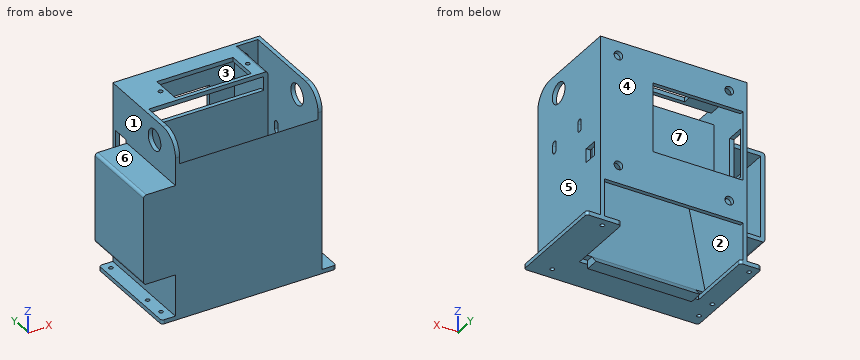
from build123d import *

# Parameters (mm, degrees)
SKETCH_1_W                      = 126
SKETCH_1_H                      = 75
EXTRUDE_1_DEPTH                 = 3
CUT_EXTRUDE_2_REACH             = 148.663
SKETCH_3_W                      = 86
SKETCH_3_H                      = 50
SKETCH_2_R                      = 1.5
CUT_EXTRUDE_1_DEPTH             = 147.662878739
SKETCH_4_W                      = 3
SKETCH_4_H                      = 75
EXTRUDE_2_DEPTH                 = 130
SKETCH_10_W                     = 100
SKETCH_10_H                     = 3
EXTRUDE_5_DEPTH                 = 100
CUT_EXTRUDE_5_REACH             = 199.965
SKETCH_9_R                      = 3.1
CUT_EXTRUDE_5_DIRECTION_2_DEPTH = 198.964643308
EXTRUDE_7_REACH                 = 191.955
CUT_EXTRUDE_9_DEPTH             = 190.95525789
CUT_EXTRUDE_9_DEPTH_BACK        = 190.95525789
SKETCH_18_R                     = 7.55
SKETCH_33_W                     = 65
SKETCH_33_H                     = 50
CUT_EXTRUDE_14_DEPTH            = 5
FILLET_1_R                      = 2
FILLET_2_R                      = 15
CUT_EXTRUDE_11_DEPTH            = 10
SKETCH_37_W                     = 89
SKETCH_37_H                     = 75
SKETCH_37_W_2                   = 83
SKETCH_37_H_2                   = 69
EXTRUDE_21_DEPTH                = 35
EXTRUDE_22_REACH                = 191.955
SKETCH_38_W                     = 59
SKETCH_38_H                     = 3
EXTRUDE_START                   = 5
EXTRUDE_23_DEPTH                = 75
SKETCH_43_W                     = 65
SKETCH_43_H                     = 58
EXTRUDE_24_DEPTH                = 23
SKETCH_44_W                     = 20
SKETCH_44_H                     = 59
CUT_EXTRUDE_15_DEPTH            = 55
SKETCH_48_W                     = 35
SKETCH_48_H                     = 13
CUT_EXTRUDE_16_DEPTH            = 12
SKETCH_49_W                     = 55
SKETCH_49_H                     = 22
CUT_EXTRUDE_18_DEPTH            = 12
SKETCH_50_R                     = 1.6
SKETCH_50_R_2                   = 1.5
CUT_EXTRUDE_19_DEPTH            = 12
CUT_EXTRUDE_21_REACH            = 201.887
SKETCH_52_W                     = 10
SKETCH_52_H                     = 10
FILLET_3_R                      = 2
SKETCH_53_W                     = 100
SKETCH_53_H                     = 3
EXTRUDE_25_DEPTH                = 3


with BuildPart() as part:
    # 草图1 → 凸台-拉伸1 (new body)
    with BuildSketch(Plane.XY):
        with Locations((63, 37.5)):
            Rectangle(SKETCH_1_W, SKETCH_1_H)
    extrude(amount=EXTRUDE_1_DEPTH)

    # 草图3 → 切除-拉伸2 (cut, up to next)
    with BuildSketch(Plane(origin=(0, 0, 0), x_dir=(-1, 0, 0), z_dir=(0, 0, -1)), mode=Mode.PRIVATE) as cut_extrude_2_sk1:
        with Locations((-58, 50)):
            Rectangle(SKETCH_3_W, SKETCH_3_H)
    cut_extrude_2_tool1 = extrude(cut_extrude_2_sk1.sketch, amount=-CUT_EXTRUDE_2_REACH, mode=Mode.PRIVATE) & part.part
    add(cut_extrude_2_tool1.solids().sort_by_distance((58, 50, 0))[0], mode=Mode.SUBTRACT)

    # 草图2 → 切除-拉伸1 (cut, through all)
    with BuildSketch(Plane.XY.offset(3)):
        with Locations((5, 69)):
            Circle(SKETCH_2_R)
        with Locations((5, 25)):
            Circle(SKETCH_2_R)
        with Locations((5, 9)):
            Circle(SKETCH_2_R)
        with Locations((111, 69)):
            Circle(SKETCH_2_R)
        with Locations((111, 9)):
            Circle(SKETCH_2_R)
    extrude(amount=-CUT_EXTRUDE_1_DEPTH, mode=Mode.SUBTRACT)

    # 草图4 → 凸台-拉伸2 (add)
    with BuildSketch(Plane.XY.offset(3)):
        with Locations((11.5, 37.5)):
            Rectangle(SKETCH_4_W, SKETCH_4_H)
    extrude_2 = extrude(amount=EXTRUDE_2_DEPTH)

    # 镜向1: 凸台-拉伸2 across plane
    add(extrude_2.mirror(Plane.ZY.offset(-63)))

    # 草图10 → 凸台-拉伸5 (add)
    with BuildSketch(Plane(origin=(13, 0, 0), x_dir=(0, 0, -1), z_dir=(1, 0, 0))):
        with Locations((-83, 73.5)):
            Rectangle(SKETCH_10_W, SKETCH_10_H)
    extrude(amount=EXTRUDE_5_DEPTH)

    # 草图9 → 切除-拉伸5 (cut, up to next)
    with BuildSketch(Plane(origin=(0, 75, 0), x_dir=(1, 0, 0), z_dir=(0, 1, 0)), mode=Mode.PRIVATE) as cut_extrude_5_sk1:
        with Locations(Location((23, -123, 0), (0, 0, 180))):
            Circle(SKETCH_9_R)
    cut_extrude_5_tool1 = extrude(cut_extrude_5_sk1.sketch, amount=-CUT_EXTRUDE_5_REACH, mode=Mode.PRIVATE) & part.part
    # 草图9 → 切除-拉伸5 (cut, up to next)
    with BuildSketch(Plane(origin=(0, 75, 0), x_dir=(1, 0, 0), z_dir=(0, 1, 0)), mode=Mode.PRIVATE) as cut_extrude_5_sk2:
        with Locations(Location((23, -43, 0), (0, 0, 180))):
            Circle(SKETCH_9_R)
    cut_extrude_5_tool2 = extrude(cut_extrude_5_sk2.sketch, amount=-CUT_EXTRUDE_5_REACH, mode=Mode.PRIVATE) & part.part
    # 草图9 → 切除-拉伸5 (cut, up to next)
    with BuildSketch(Plane(origin=(0, 75, 0), x_dir=(1, 0, 0), z_dir=(0, 1, 0)), mode=Mode.PRIVATE) as cut_extrude_5_sk3:
        with Locations(Location((103, -123, 0), (0, 0, 180))):
            Circle(SKETCH_9_R)
    cut_extrude_5_tool3 = extrude(cut_extrude_5_sk3.sketch, amount=-CUT_EXTRUDE_5_REACH, mode=Mode.PRIVATE) & part.part
    # 草图9 → 切除-拉伸5 (cut, up to next)
    with BuildSketch(Plane(origin=(0, 75, 0), x_dir=(1, 0, 0), z_dir=(0, 1, 0)), mode=Mode.PRIVATE) as cut_extrude_5_sk4:
        with Locations(Location((103, -43, 0), (0, 0, 180))):
            Circle(SKETCH_9_R)
    cut_extrude_5_tool4 = extrude(cut_extrude_5_sk4.sketch, amount=-CUT_EXTRUDE_5_REACH, mode=Mode.PRIVATE) & part.part
    add(cut_extrude_5_tool1.solids().sort_by_distance((23, 75, 123))[0], mode=Mode.SUBTRACT)
    add(cut_extrude_5_tool2.solids().sort_by_distance((23, 75, 43))[0], mode=Mode.SUBTRACT)
    add(cut_extrude_5_tool3.solids().sort_by_distance((103, 75, 123))[0], mode=Mode.SUBTRACT)
    add(cut_extrude_5_tool4.solids().sort_by_distance((103, 75, 43))[0], mode=Mode.SUBTRACT)

    # 草图9 → 切除-拉伸5 direction 2 (cut)
    with BuildSketch(Plane(origin=(0, 75, 0), x_dir=(1, 0, 0), z_dir=(0, 1, 0))):
        with Locations(Location((23, -123, 0), (0, 0, 180))):
            Circle(SKETCH_9_R)
        with Locations(Location((23, -43, 0), (0, 0, 180))):
            Circle(SKETCH_9_R)
        with Locations(Location((103, -123, 0), (0, 0, 180))):
            Circle(SKETCH_9_R)
        with Locations(Location((103, -43, 0), (0, 0, 180))):
            Circle(SKETCH_9_R)
    extrude(amount=CUT_EXTRUDE_5_DIRECTION_2_DEPTH, mode=Mode.SUBTRACT)

    # 凸台-拉伸7: up to this face of the body (flat: up to its plane)
    extrude_7_end = Plane(part.part.faces().sort_by_distance((113, 36.357142857, 67.523809524))[0])
    # 草图17 → 凸台-拉伸7 (add, up to the picked face)
    with BuildSketch(Plane(origin=(13, 0, 0), x_dir=(0, 0, -1), z_dir=(1, 0, 0)), mode=Mode.PRIVATE) as extrude_7_sk1:
        Polygon((-3, 0), (-113, 0), (-3, 30), align=None)
    extrude_7_tool1 = split(extrude(extrude_7_sk1.sketch, amount=EXTRUDE_7_REACH, mode=Mode.PRIVATE), bisect_by=extrude_7_end, keep=Keep.BOTH, mode=Mode.PRIVATE)
    add(extrude_7_tool1.solids().sort_by(Axis((13, 10, 39.666667), (1, 0, 0)))[0])

    # 草图18 → 切除-拉伸9 (cut, two sides: drawn at the far end of the back side and taken through both)
    with BuildSketch(Plane(origin=(13, 0, 0), x_dir=(0, 0, -1), z_dir=(1, 0, 0)).offset(-CUT_EXTRUDE_9_DEPTH_BACK)):
        with Locations(Location((-118, 25, 0), (0, 0, 90))):
            Circle(SKETCH_18_R)
    extrude(amount=CUT_EXTRUDE_9_DEPTH + CUT_EXTRUDE_9_DEPTH_BACK, mode=Mode.SUBTRACT)

    # 草图33 → 切除-拉伸14 (cut)
    with BuildSketch(Plane(origin=(0, 75, 0), x_dir=(1, 0, 0), z_dir=(0, 1, 0))):
        with Locations((45.5, -86)):
            Rectangle(SKETCH_33_W, SKETCH_33_H)
    extrude(amount=-CUT_EXTRUDE_14_DEPTH, mode=Mode.SUBTRACT)

    # 圆角1
    fillet_1_edges = [part.edges().sort_by_distance(p)[0] for p in [
        (101, 75, 1.5),
        (15, 75, 1.5),
        (0, 0, 1.5),
        (0, 75, 1.5),
        (126, 75, 1.5),
        (126, 0, 1.5),
    ]]
    fillet(fillet_1_edges, radius=FILLET_1_R)

    # 圆角2
    fillet_2_edges = [part.edges().sort_by_distance(p)[0] for p in [
        (11.5, 0, 133),
        (114.5, 0, 133),
    ]]
    fillet(fillet_2_edges, radius=FILLET_2_R)

    # 草图20 → 切除-拉伸11 (cut)
    with BuildSketch(Plane(origin=(116, 0, 0), x_dir=(0, 0, -1), z_dir=(1, 0, 0))):
        with BuildLine():
            Line((-83.606081957, 51.95), (-78.606081957, 51.95))
            ThreePointArc((-78.606081957, 51.95), (-76.556081957, 49.9), (-78.606081957, 47.85))
            Line((-78.606081957, 47.85), (-83.606081957, 47.85))
            ThreePointArc((-83.606081957, 47.85), (-85.656081957, 49.9), (-83.606081957, 51.95))
        make_face()
        with BuildLine():
            Line((-83.606081957, 21.95), (-78.606081957, 21.95))
            ThreePointArc((-78.606081957, 21.95), (-76.556081957, 19.9), (-78.606081957, 17.85))
            Line((-78.606081957, 17.85), (-83.606081957, 17.85))
            ThreePointArc((-83.606081957, 17.85), (-85.656081957, 19.9), (-83.606081957, 21.95))
        make_face()
    extrude(amount=-CUT_EXTRUDE_11_DEPTH, mode=Mode.SUBTRACT)

    # 草图37 → 凸台-拉伸21 (add)
    with BuildSketch(Plane.XZ.offset(-72)):
        with Locations((54.5, 95.5)):
            Rectangle(SKETCH_37_W, SKETCH_37_H)
        with Locations((54.5, 95.5)):
            Rectangle(SKETCH_37_W_2, SKETCH_37_H_2, mode=Mode.SUBTRACT)
    extrude(amount=EXTRUDE_21_DEPTH)

    # 草图38 → 凸台-拉伸22 (add, up to next)
    with BuildSketch(Plane(origin=(13, 0, 0), x_dir=(0, 0, -1), z_dir=(1, 0, 0)), mode=Mode.PRIVATE) as extrude_22_sk1:
        with Locations((-90.5, 38.5)):
            Rectangle(SKETCH_38_W, SKETCH_38_H)
    extrude_22_tool1 = extrude(extrude_22_sk1.sketch, amount=EXTRUDE_22_REACH, mode=Mode.PRIVATE) - part.part
    add(extrude_22_tool1.solids().sort_by_distance((13, 38.5, 90.5))[0])

    # 草图41 → 凸台-拉伸23 (add)
    with BuildSketch(Plane(origin=(15, 0, 0), x_dir=(0, 0, -1), z_dir=(1, 0, 0)).offset(EXTRUDE_START)):
        Polygon((-3, 25), (-3, 30), (3, 35), (3, 25), align=None)
    extrude(amount=EXTRUDE_23_DEPTH)

    # 草图43 → 凸台-拉伸24 (add)
    with BuildSketch(Plane.ZY.offset(-10)):
        with Locations((65.5, 29)):
            Rectangle(SKETCH_43_W, SKETCH_43_H)
    extrude(amount=EXTRUDE_24_DEPTH)

    # 草图44 → 切除-拉伸15 (cut)
    with BuildSketch(Plane(origin=(0, 58, 0), x_dir=(1, 0, 0), z_dir=(0, 1, 0))):
        with Locations((0, -65.5)):
            Rectangle(SKETCH_44_W, SKETCH_44_H)
    extrude(amount=-CUT_EXTRUDE_15_DEPTH, mode=Mode.SUBTRACT)

    # 草图48 → 切除-拉伸16 (cut)
    with BuildSketch(Plane.ZY.offset(-10)):
        with Locations((82.5, 65.5)):
            Rectangle(SKETCH_48_W, SKETCH_48_H)
    extrude(amount=-CUT_EXTRUDE_16_DEPTH, mode=Mode.SUBTRACT)

    # 草图49 → 切除-拉伸18 (cut)
    with BuildSketch(Plane.XY.offset(133)):
        with Locations((61.5, 51)):
            Rectangle(SKETCH_49_W, SKETCH_49_H)
    extrude(amount=-CUT_EXTRUDE_18_DEPTH, mode=Mode.SUBTRACT)

    # 草图50 → 切除-拉伸19 (cut)
    with BuildSketch(Plane.XY.offset(133)):
        with Locations((30, 51)):
            Circle(SKETCH_50_R)
        with Locations((93, 51)):
            Circle(SKETCH_50_R_2)
    extrude(amount=-CUT_EXTRUDE_19_DEPTH, mode=Mode.SUBTRACT)

    # 草图52 → 切除-拉伸21 (cut, up to next)
    with BuildSketch(Plane(origin=(116, 0, 0), x_dir=(0, 0, -1), z_dir=(1, 0, 0)), mode=Mode.PRIVATE) as cut_extrude_21_sk1:
        with Locations((-55, 63)):
            Rectangle(SKETCH_52_W, SKETCH_52_H)
    cut_extrude_21_tool1 = extrude(cut_extrude_21_sk1.sketch, amount=-CUT_EXTRUDE_21_REACH, mode=Mode.PRIVATE) & part.part
    add(cut_extrude_21_tool1.solids().sort_by_distance((116, 63, 55))[0], mode=Mode.SUBTRACT)

    # 圆角3
    fillet_3_edges = [part.edges().sort_by_distance(p)[0] for p in [
        (99, 54.5, 133),
        (99, 54.5, 58),
        (-13, 29, 33),
        (-13, 29, 98),
    ]]
    fillet(fillet_3_edges, radius=FILLET_3_R)

    # 草图53 → 凸台-拉伸25 (add)
    with BuildSketch(Plane(origin=(0, 0, 33), x_dir=(-1, 0, 0), z_dir=(0, 0, -1))):
        with Locations((-63, 73.5)):
            Rectangle(SKETCH_53_W, SKETCH_53_H)
    extrude(amount=EXTRUDE_25_DEPTH)


solid = part.part
The listing builds one solid part. Answer for the finished solid, in the listing's coordinates (mm). Face numbers are marked on the shaded views. A direction names the side the tool comes from. Give positions to 0.01 mm unless a question says otherwise; leave off trailing zeros. Write each loop counter-clockwise with the first axis right and the second up, starting at its lowest first coordinate (ties: lowest second). Pieces come first, ordered by that corner, then holes. Notation, with made-up numbers: (6, 80.25) -> (18, 80.25) arc R16 cw to (18, 108.25) -> close; hole circle Ø3 at (30, -14.5). An arc over 180 degrees is marked (long way). One line per question, with ' | ' between items. Start each with the question number.
1. For the marked faces 5, 6 and 7, determine the directions among +Z, -Z, +X, -X, +Y, -Y from which every point of the face is accessible in a straight line to the end or side of a thin tool.
2. Section C-C (y = 19.9) is taken. State how many separate pieces and enclosed holes the cut face has, plus the area to 3 significant figures.
3. Given pin 1 Ø3.5 at (x, z) = (98.5, 1.5) entering from +Y; pin 2 Ø8 at (x, z) = (80, 18) entering from +Y; pin 3 Ø5 at (x, z) = (60.5, 97) entering from +Y, each flat-ended and moving along its own axis, determine where each tip first touches the part or whether it passes through.
4. Section D-D (x = 85.5) is taken. Determine the outline of the cut face in (y, z), plus the area to 3 significant figures.
5. Section B-B (x = 23) is taken. Determine the outline of the cut face in (y, z).
6. Find the intervals of material crossed by probe 1 along X at (y, z) = (34, 56); probe 2 along Z at (x, y) = (103, 73.8); probe 3 along X at (y, z) = (55, 119), in increasing order.
7. Section A-A (z = 69) is taken. Determine the outline of the cut face in (x, y).
8. For a pull along Y with two mould halves and no side action, classify the marked faces 1, 2, 3 and 4 as pulls with the +Y half, pulls with the -Y half, needs draft (parallel to the pull), parting line crosses it, or undercut.
Response values:
1) face 5: +Z, +X, +Y, -Y | face 6: +Z, -X, +Y, -Y | face 7: none
2) separate pieces: 4 | enclosed holes: 1 | area: 5,080 mm2
3) pin 1: y = 30 | pin 2: y = 27 | pin 3: y = 40
4) outline: (0, 0) -> (25, 0) -> (25, -3) -> (35, -3) -> (30, 3) -> (0, 113) -> close; (37, 58) -> (72, 58) -> (72, 30) -> (75, 30) -> (75, 133) -> (62, 133) -> (62, 130) -> (72, 130) -> (72, 61) -> (40, 61) -> (40, 120) -> (37, 120) -> close; (37, 130) -> (40, 130) -> (40, 133) -> (37, 133) -> close | area: 2,400 mm2
5) outline: (0, 0) -> (25, 0) -> (25, -3) -> (35, -3) -> (30, 3) -> (0, 113) -> close; (37, 58) -> (72, 58) -> (72, 46.1) -> (75, 46.1) -> (75, 61) -> (40, 61) -> (40, 120) -> (37, 120) -> close; (37, 130) -> (72, 130) -> (72, 126.1) -> (75, 126.1) -> (75, 133) -> (37, 133) -> close; (72, 30) -> (75, 30) -> (75, 39.9) -> (72, 39.9) -> close; (72, 111) -> (75, 111) -> (75, 119.9) -> (72, 119.9) -> close
6) probe 1: -13 to -10, 10 to 13, 113 to 116 | probe 2: 0 to 3, 30 to 39.9, 46.1 to 119.9, 126.1 to 133 | probe 3: 10 to 13, 96 to 99, 113 to 116
7) outline: (-13, 0) -> (116, 0) -> (116, 75) -> (78, 75) -> (78, 72) -> (96, 72) -> (96, 40) -> (13, 40) -> (13, 59) -> (10, 59) -> (10, 3) -> (-10, 3) -> (-10, 58) -> (-13, 58) -> close; (10, 72) -> (13, 72) -> (13, 75) -> (10, 75) -> close; hole (13, 12) -> (113, 12) -> (113, 72) -> (99, 72) -> (99, 37) -> (13, 37) -> close
8) face 1: needs draft | face 2: undercut | face 3: undercut | face 4: pulls with the +Y half
